from build123d import *

# Parameters (mm, degrees)
SKETCH1_W               = 25
SKETCH1_H               = 38
BOSS_EXTRUDE1_DEPTH     = 5
SKETCH4_R               = 4.15
CUT_EXTRUDE2_DEPTH      = 6
SKETCH9_W               = 17.7
SKETCH9_H               = 31.6
BOSS_EXTRUDE3_DEPTH     = 2.8
SKETCH6_R               = 1.6
CUT_EXTRUDE4_DEPTH      = 3.8
CUT_EXTRUDE4_DEPTH_BACK = 6
CHAMFER1_SIZE           = 1
CHAMFER1_SIZE2          = 0.577350269
CHAMFER1_PART_2_SIZE    = 1
CHAMFER1_PART_2_SIZE2   = 0.577350269
CHAMFER1_PART_3_SIZE    = 1
CHAMFER1_PART_3_SIZE2   = 0.577350269
CHAMFER1_PART_4_SIZE    = 1
CHAMFER1_PART_4_SIZE2   = 0.577350269
SKETCH10_R              = 4.15
BOSS_EXTRUDE4_DEPTH     = 5


with BuildPart() as part:
    # Sketch1 → Boss-Extrude1 (new body)
    with BuildSketch(Plane(origin=(0, 0, 0), x_dir=(1, 0, 0), z_dir=(0, 1, 0))):
        Rectangle(SKETCH1_W, SKETCH1_H)
    extrude(amount=BOSS_EXTRUDE1_DEPTH)

    # Sketch4 → Cut-Extrude2 (cut, through all)
    with BuildSketch(Plane(origin=(0, 5, 0), x_dir=(1, 0, 0), z_dir=(0, 1, 0))):
        Circle(SKETCH4_R)
    extrude(amount=-CUT_EXTRUDE2_DEPTH, mode=Mode.SUBTRACT)

    # Sketch9 → Boss-Extrude3 (add)
    with BuildSketch(Plane(origin=(0, 5, 0), x_dir=(1, 0, 0), z_dir=(0, 1, 0))):
        Rectangle(SKETCH9_W, SKETCH9_H)
    extrude(amount=BOSS_EXTRUDE3_DEPTH)

    # Sketch6 → Cut-Extrude4 (cut, two sides)
    with BuildSketch(Plane(origin=(0, 5, 0), x_dir=(1, 0, 0), z_dir=(0, 1, 0))) as cut_extrude4_sk:
        with Locations((9, -16)):
            Circle(SKETCH6_R)
        with Locations((-9, -16)):
            Circle(SKETCH6_R)
        with Locations((-9, 16)):
            Circle(SKETCH6_R)
        with Locations((9, 16)):
            Circle(SKETCH6_R)
    extrude(amount=CUT_EXTRUDE4_DEPTH, mode=Mode.SUBTRACT)
    extrude(cut_extrude4_sk.sketch, amount=-CUT_EXTRUDE4_DEPTH_BACK, mode=Mode.SUBTRACT)

    # Chamfer1
    chamfer1_edges = [part.edges().sort_by_distance(p)[0] for p in [
        (8.85, 7.8, 0),
    ]]
    chamfer1_side = [part.faces().sort_by_distance(p)[0] for p in [
        (8.85, 6.4, 0),
    ]]
    chamfer(chamfer1_edges, length=CHAMFER1_SIZE, length2=CHAMFER1_SIZE2, reference=chamfer1_side[0])

    # Chamfer1 part 2
    chamfer1_part_2_edges = [part.edges().sort_by_distance(p)[0] for p in [
        (0, 7.8, 15.8),
    ]]
    chamfer1_part_2_side = [part.faces().sort_by_distance(p)[0] for p in [
        (0, 6.4, 15.8),
    ]]
    chamfer(chamfer1_part_2_edges, length=CHAMFER1_PART_2_SIZE, length2=CHAMFER1_PART_2_SIZE2, reference=chamfer1_part_2_side[0])

    # Chamfer1 part 3
    chamfer1_part_3_edges = [part.edges().sort_by_distance(p)[0] for p in [
        (0, 7.8, -15.8),
    ]]
    chamfer1_part_3_side = [part.faces().sort_by_distance(p)[0] for p in [
        (0, 6.4, -15.8),
    ]]
    chamfer(chamfer1_part_3_edges, length=CHAMFER1_PART_3_SIZE, length2=CHAMFER1_PART_3_SIZE2, reference=chamfer1_part_3_side[0])

    # Chamfer1 part 4
    chamfer1_part_4_edges = [part.edges().sort_by_distance(p)[0] for p in [
        (-8.85, 7.8, 0),
    ]]
    chamfer1_part_4_side = [part.faces().sort_by_distance(p)[0] for p in [
        (-8.85, 6.4, 0),
    ]]
    chamfer(chamfer1_part_4_edges, length=CHAMFER1_PART_4_SIZE, length2=CHAMFER1_PART_4_SIZE2, reference=chamfer1_part_4_side[0])

    # Sketch10 → Boss-Extrude4 (add)
    with BuildSketch(Plane.XZ.offset(-5)):
        Circle(SKETCH10_R)
    extrude(amount=BOSS_EXTRUDE4_DEPTH)


solid = part.part
Check sheet for the modelled part. Datum: model origin and axes. Units: mm. A direction names the side the tool comes from. Round coordinates to 2 decimals unless told otherwise and drop trailing zeros. Order: outer loops, then holes, each group sorted by start corner. A loop starts at its lowest first (then second) coordinate and runs counter-clockwise, first axis right, second up.
Q1. Scan lines: L1, parallel to Z at x = -9, y = 3.5; L2, parallel to X at y = 4, z = 16; L3, parallel to Y at x = -10, z = 2.5. Record each from-to range of solid material in increasing order.
Filled sheet:
L1: z = -19 to -17.6, -14.4 to 14.4, 17.6 to 19
L2: x = -12.5 to -10.6, -7.4 to 7.4, 10.6 to 12.5
L3: y = 0 to 5
Q2. Cross-section at D-D, the plane x = -2.75. Enter the section's corners in (y, z), plus the area to 3 significant figures.
Filled sheet:
outline: (0, -19) - (5, -19) - (5, -15.8) - (6.8, -15.8) - (7.8, -15.22) - (7.8, 15.22) - (6.8, 15.8) - (5, 15.8) - (5, 19) - (0, 19) - close
area: 278 mm2
Q3. Cross-section at B-B, the plane z = 4.5. Enter the section's corners in (x, y).
Filled sheet:
outline: (-12.5, 0) - (12.5, 0) - (12.5, 5) - (8.85, 5) - (8.85, 6.8) - (8.27, 7.8) - (-8.27, 7.8) - (-8.85, 6.8) - (-8.85, 5) - (-12.5, 5) - close
Q4. Cross-section at A-A, the plane y = 6.25. Enter the section's corners in (x, z).
Filled sheet:
outline: (-8.85, -14.41) arc R1.6 cw to (-7.41, -15.8) - (7.41, -15.8) arc R1.6 cw to (8.85, -14.41) - (8.85, 14.41) arc R1.6 cw to (7.41, 15.8) - (-7.41, 15.8) arc R1.6 cw to (-8.85, 14.41) - close
Q5. Depth check by flat-ended pin: P1, Ø0.5, axis at x = 0.5, y = 6, coming from the +Z side; P2, Ø0.5, axis at y = 6, z = 1.5, coming from the +X side; P3, Ø1.4, axis at x = 2, y = 6, coming from the -Z side. Enter the tip coordinate at first touch or a pass-through.
Filled sheet:
P1: stops at z = 15.8
P2: stops at x = 8.85
P3: stops at z = -15.8
Q6. Draft check along Z on faces 1 (the face through (0, 2, -19)), 2 (the face through (0, 0, 0)), 3 (the face through (-8.26, 3.09, -14.58)), 4 (the face through (7.82, 3.09, 14.92)). Enter one of: pulls with the +Z half, pulls with the -Z half, needs draft (parallel to the pull), parting line crosses it, or undercut.
Filled sheet:
face 1: pulls with the -Z half
face 2: needs draft
face 3: undercut
face 4: undercut
Q7. Set-up check for faces 5 (the face through (0, 6, -15.8)), 6 (the face through (8.85, 6, 0)), 7 (the face through (-8.85, 6, 0)): record each of +Z, -Z, +X, -X, +Y, -Y from which the full face is reachable in a straight line by a thin tool's end or side.
Filled sheet:
face 5: -Z, +X, -X, +Y
face 6: +Z, -Z, +X, +Y
face 7: +Z, -Z, -X, +Y
Q8. Cross-section at C-C, the plane y = 1.5. Enter the section's corners in (x, z), plus the area to 3 significant figures.
Filled sheet:
outline: (-12.5, -19) - (12.5, -19) - (12.5, 19) - (-12.5, 19) - close; hole circle Ø3.2 at (-9, -16); hole circle Ø3.2 at (-9, 16); hole circle Ø3.2 at (9, -16); hole circle Ø3.2 at (9, 16)
area: 918 mm2
